For this review, use the dimensioned drawing (mm, ordinates from the lowest corner) and the shaded views. A direction names the side the tool comes from. Give positions to 0.01 mm unless a question says otherwise; leave off trailing zeros. Write each loop counter-clockwise with the first axis right and the second up, starting at its lowest first coordinate (ties: lowest second). Pieces come first, ordered by that corner, then holes. Notation, with made-up numbers: M -31,54 L 11,54 A8 cw 11,66 Z; hole C 48,25 d8. An arc over 180 degrees is marked long. Answer in a Markdown table with one row per item.
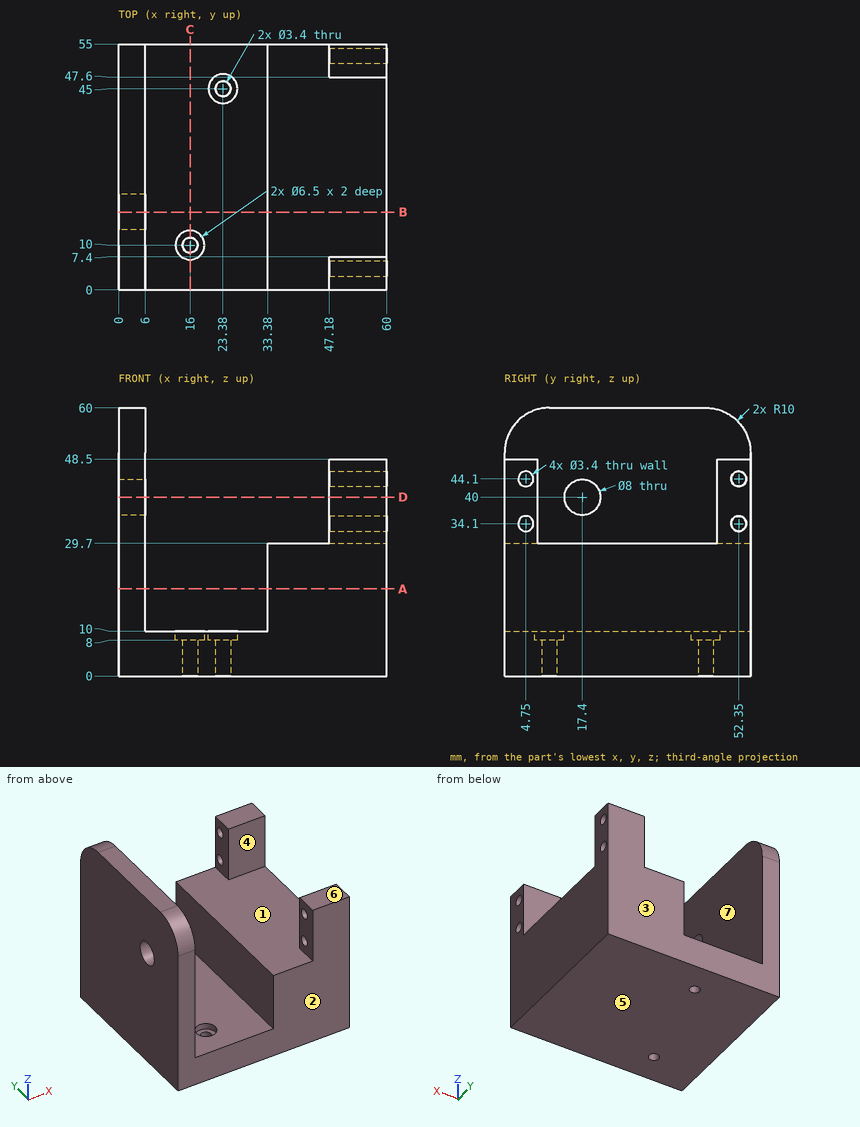
1) Add section B-B (y = 17.4). Write out the cut boundary in (x, z).
Geometry says:
| item | result |
|---|---|
| outline | M 0,0 L 60,0 L 60,29.7 L 33.38,29.7 L 33.38,10 L 6,10 L 6,36 L 0,36 Z; M 0,44 L 6,44 L 6,60 L 0,60 Z |
2) Insertion check: P1, Ø3, axis at x = 15, y = 9.5, coming from the +Z side; P2, Ø3, axis at x = 16, y = 10, coming from the +Z side; P3, Ø8.5, axis at x = 16, y = 10, coming from the +Z side; P4, Ø6, axis at x = 54, y = 50.5, coming from the +Z side. Each pin has a flat end and moves straight along its axis. Give the tip position at first contact, or say it passes through.
Geometry says:
| item | result |
|---|---|
| P1 | z = 8 |
| P2 | through |
| P3 | z = 10 |
| P4 | z = 48.5 |
3) For the marked faces 4, 5, 6 and 7, list the 3-axis set-ups (+Z, -Z, +X, -X, +Y, -Y) from which the entire face can be reached by the end or side of a thin tool; tool diameter is ignored.
Geometry says:
| item | result |
|---|---|
| face 4 | +Z, +X |
| face 5 | -Z, +X, -X, +Y, -Y |
| face 6 | +Z, +X, +Y, -Y |
| face 7 | +Z, +Y, -Y |
4) Add section A-A (z = 19.5). Write out the cut boundary in (x, y).
Geometry says:
| item | result |
|---|---|
| outline | M 0,0 L 6,0 L 6,55 L 0,55 Z; M 33.38,0 L 60,0 L 60,55 L 33.38,55 Z |
5) Add section D-D (z = 40). Write out the cut boundary in (x, y), and give its area (3 significant figures).
Geometry says:
| item | result |
|---|---|
| outline | M 0,0 L 6,0 L 6,13.4 L 0,13.4 Z; M 0,21.4 L 6,21.4 L 6,55 L 0,55 Z; M 47.18,0 L 60,0 L 60,7.4 L 47.18,7.4 Z; M 47.18,47.6 L 60,47.6 L 60,55 L 47.18,55 Z |
| area | 472 mm^2 |
6) To check wall thickness, follow probe 1 along X at (y, z) = (9.5, 12); probe 2 along X at (y, z) = (49, 36); probe 3 along Y at (x, z) = (16, 3.75). State the ranges of each line that lie inside material, in increasing order. Write a range as [from, to].
Geometry says:
| item | result |
|---|---|
| probe 1 | [0, 6], [33.38, 60] |
| probe 2 | [0, 6], [47.18, 60] |
| probe 3 | [0, 8.3], [11.7, 55] |
7) The part is to be moulded in two halves that separate along Y. For the marked faces 1, 2 and 3, say which applies: released by +Y, released by -Y, zero draft, split by the parting line, or undercut.
Geometry says:
| item | result |
|---|---|
| face 1 | undercut |
| face 2 | released by -Y |
| face 3 | released by +Y |
8) Add section C-C (x = 16). Write out the cut boundary in (y, z).
Geometry says:
| item | result |
|---|---|
| outline | M 0,0 L 8.3,0 L 8.3,8 L 6.75,8 L 6.75,10 L 0,10 Z; M 11.7,0 L 55,0 L 55,10 L 13.25,10 L 13.25,8 L 11.7,8 Z |
